For this review, take the finished solid that the model builds, in its own axes (mm). Round coordinates to 2 decimals unless told otherwise and drop trailing zeros. Order: outer loops, then holes, each group sorted by start corner. A loop starts at its lowest first (then second) coordinate and runs counter-clockwise, first axis right, second up. Notation, with made-up numbers: M 7,17.25 L 17,17.25 A27 cw 17,42.25 Z; hole C 72,-18 d5. An arc over 180 degrees is marked long. Answer in a Markdown table with one row per item. Add a question column.
```python
from build123d import *

# Parameters (mm, degrees)
F1_DEPTH = 127
F2_R     = 12.7
F3_R     = 5.08


with BuildPart() as f1:
    # F0 (on Front) → F1 (new body)
    with BuildSketch(Plane.XZ):
        Polygon((-41.956668, 44.650039), (-41.956668, 0), (29.74316, 0), (-3.856668, 44.650039), align=None)
    extrude(amount=F1_DEPTH)

    # F2
    f2_edges = [f1.edges().sort_by_distance(p)[0] for p in [
        (-3.856668, -63.5, 44.650039),
    ]]
    fillet(f2_edges, radius=F2_R)

    # F3
    f3_edges = [f1.edges().sort_by_distance(p)[0] for p in [
        (-26.07529, -127, 44.650039),
        (-4.523432, -127, 43.313826),
        (-41.956668, -127, 22.325019),
        (14.848492, -127, 19.793182),
        (-6.106754, -127, 0),
        (-41.956668, -63.5, 44.650039),
    ]]
    fillet(f3_edges, radius=F3_R)


solid = f1.part
```
1. To check wall thickness, follow probe 1 along X at (y, z) = (-107.5, 39.5); probe 2 along X at (y, z) = (-116, 35.5); probe 3 along Z at (x, y) = (-9.5, -15.5). State the ranges of each line that lie inside material, in increasing order. Write a range as [from, to].
2. Consider section A-A on y = -39.5. Write out the cut boundary in (x, z), plus the area to 3 significant figures.
3. Clearance check with flat-ended pins moving along their axes: pin 1 Ø4 at (y, z) = (-39.5, 33.5) entering from +X; pin 2 Ø3 at (y, z) = (-18.5, 16) entering from +X. State where each tip first meets the part, or that it passes through.
Solved:
| question | item | result |
|---|---|---|
| 1 | probe 1 | x = [-41.96, 0.02] |
| 1 | probe 2 | x = [-41.96, 3.03] |
| 1 | probe 3 | z = [0, 44.63] |
| 2 | outline | M -41.96,0 L 29.74,0 L -0.05,39.59 A12.7 ccw -10.19,44.65 L -36.88,44.65 A5.08 ccw -41.96,39.57 Z |
| 2 | area | 2,440 mm^2 |
| 3 | pin 1 | stops at x = 6.04 |
| 3 | pin 2 | stops at x = 18.83 |
